Input: dimensioned drawing with shaded views. Units: mm. Origin: part minimum x, y, z. A direction names the side the tool comes from. Round coordinates to 2 decimals unless told otherwise and drop trailing zeros. Loops run counter-clockwise (first coordinate to the right, second up) from the corner with the lowest first, then second, coordinate; pieces in that order, holes last. Notation, with made-up numbers: M -30,-21.75 L 4,-21.75 A28 cw 4,4.25 Z; hole C 41,51.25 d1. An arc over 180 degrees is marked long. One line per item, written item: value.
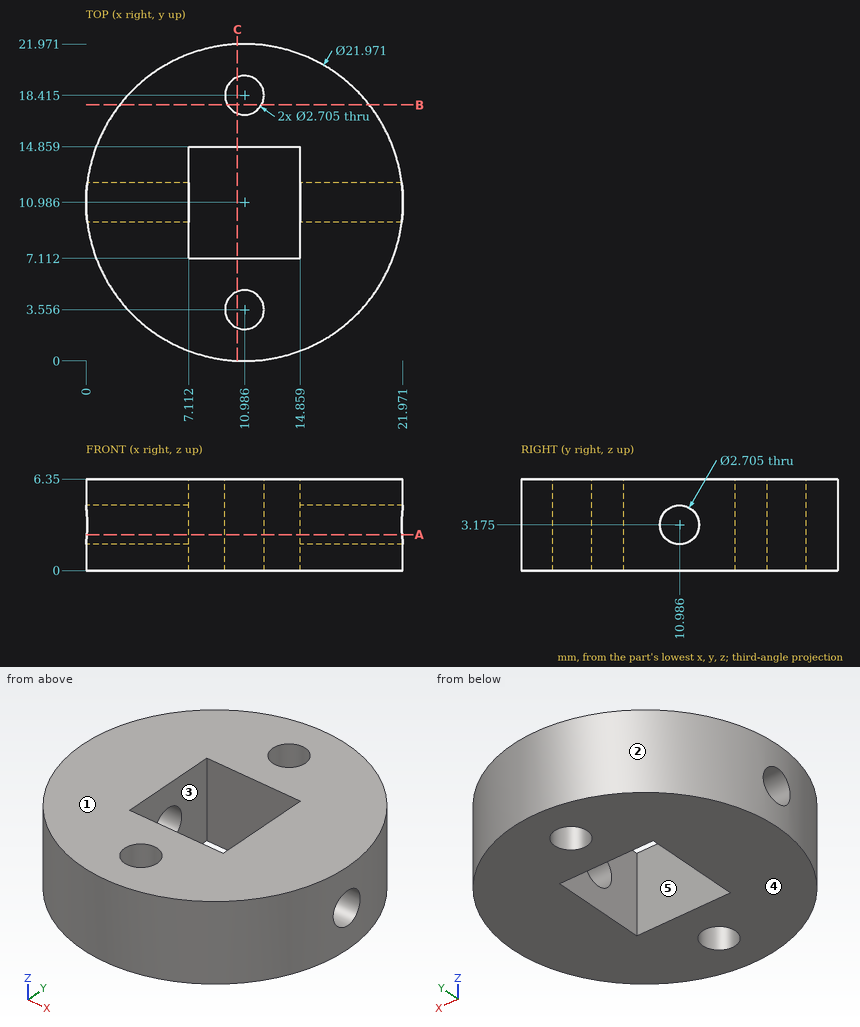
1. Section query A-A (z = 2.5). Return the cut outline in (x, y) (1 decimal).
Report:
outline: M 0.1,9.8 A11 ccw 21.9,9.8 L 14.9,9.8 L 14.9,7.1 L 7.1,7.1 L 7.1,9.8 Z; M 0.1,12.2 L 7.1,12.2 L 7.1,14.9 L 14.9,14.9 L 14.9,12.2 L 21.9,12.2 A11 ccw Z; hole C 11,3.6 d2.7; hole C 11,18.4 d2.7
2. Section query C-C (x = 10.5). Return the cut outline in (y, z).
Report:
outline: M 0.01,0 L 2.29,0 L 2.29,6.35 L 0.01,6.35 Z; M 4.82,0 L 7.11,0 L 7.11,6.35 L 4.82,6.35 Z; M 14.86,0 L 17.15,0 L 17.15,6.35 L 14.86,6.35 Z; M 19.68,0 L 21.96,0 L 21.96,6.35 L 19.68,6.35 Z
3. Ray query, line 1 (Y direction, x = 11, z = 6.25); line 2 (X direction, y = 10.25, z = 5) (1 decimal); line 3 (Y direction, x = 14, z = 5.5). Return the intervals inside material, ascending. Write a range as [from, to].
Report:
line 1: y = [0, 2.2], [4.91, 7.11], [14.86, 17.06], [19.77, 21.97]
line 2: x = [0, 7.1], [14.9, 21.9]
line 3: y = [0.42, 7.11], [14.86, 21.55]
4. Pull-direction query (Y, two-part tool) for the marked faces 1, 2 and 3; classes: released by +Y, released by -Y, zero draft, split by the parting line, or undercut.
Report:
face 1: zero draft
face 2: split by the parting line
face 3: undercut
5. Reachability of the marked faces 4 and 5 from +Z, -Z, +X, -X, +Y, -Y: full face, straight path, thin tool, end or side. Return the list, or none.
Report:
face 4: -Z, +X, -X, +Y, -Y
face 5: +Z, -Z
6. Section query B-B (y = 17.75). Return the cut outline in (x, z).
Report:
outline: M 2.33,0 L 9.81,0 L 9.81,6.35 L 2.33,6.35 Z; M 12.16,0 L 19.64,0 L 19.64,6.35 L 12.16,6.35 Z
